For this review, take the finished solid that the model builds, in its own axes (mm). Give positions to 0.01 mm unless a question says otherwise; leave off trailing zeros. Loops run counter-clockwise (first coordinate to the right, second up) from the corner with the lowest first, then second, coordinate; pieces in that order, holes last.
Autodesk Inventor part; units mm, degrees
ref_plane "YZ Plane" through (0, 0, 0) normal (1, 0, 0) x (0, 1, 0)
ref_plane "XZ Plane" through (0, 0, 0) normal (0, 1, 0) x (-1, 0, 0)
ref_plane "XY Plane" through (0, 0, 0) normal (0, 0, 1) x (1, 0, 0)
sketch "Sketch1" plane through (0, 0, 0) normal (0, 0, 1) x (1, 0, 0)
  point P0 (0, 0)
sketch "Sketch2" plane through (0, 0, 0) normal (0, 0, 1) x (1, 0, 0)
  circle A0 centre (0, 0) radius 50
  dimension "d0" = 100
extrude "Extrusion1" add sketch "Sketch2" along normal blind 10
sketch "Sketch5" plane through (0, 0, 10) normal (0, 0, 1) x (1, 0, 0)
  circle A0 centre (0, 0) radius 12.5
  line L0 (0, 0) -> (0, 36)
  circle A1 centre (0, 36) radius 4
  dimension "d16" = 36
  dimension "d17" = 8
extrude "Extrusion4" cut sketch "Sketch5" against normal blind 10 contours A1
sketch "Sketch7" plane through (0, 0, 10) normal (0, 0, 1) x (1, 0, 0)
  circle A0 centre (0, 0) radius 5.5
  dimension "d26" = 11
extrude "Extrusion6" cut sketch "Sketch7" against normal blind 10
pattern_circular "Circular Pattern2" count 6 over 360 about axis through (0, 0, 10) along (0, 0, -1) of "Extrusion4"
equation "\"BendRadius\" = Thickness"
equation "\"BendReliefWidth\" = Thickness"
equation "\"BendReliefDepth\" = 0.5 * Thickness"
equation "\"CornerReliefSize\" = 4 * Thickness"
equation "\"MinimumRemnant\" = 2 * Thickness"
equation "\"TransitionRadius\" = BendRadius"
equation "\"JacobiRadiusSize\" = BendRadius"
equation "\"GapSize\" = Thickness"
properties part number "capp"
Q1. Consider section B-B on y = 0. Give the boundary of the cut face in (x, z).
Answers:
outline: (-50, 0) - (-5.5, 0) - (-5.5, 10) - (-50, 10) - close; (5.5, 0) - (50, 0) - (50, 10) - (5.5, 10) - close
Q2. Mouldability with a two-part tool opening along X and no side actions: class faces 1 (the cylindrical face through (-29.33, -21.55, 5.07)), 2 (the cylindrical face through (47.69, -15.02, 4.93)), 3 (the flat face through (-1, -10, 0)), 4 (the cylindrical face through (-1.19, -5.37, 5.07)) as +X half, -X half, draft (parallel to the pull), parting line (faces both ways), or undercut.
Answers:
face 1: undercut
face 2: parting line
face 3: draft
face 4: undercut
Q3. Consider section C-C on y = 19. Give the boundary of the cut face in (x, z).
Answers:
outline: (-46.25, 0) - (-35.05, 0) - (-35.05, 10) - (-46.25, 10) - close; (-27.3, 0) - (27.3, 0) - (27.3, 10) - (-27.3, 10) - close; (35.05, 0) - (46.25, 0) - (46.25, 10) - (35.05, 10) - close
Q4. For pin 1 Ø7 at (x, y) = (0, 36) entering from -Z; pin 2 Ø14.5 at (x, y) = (0, 0) entering from -Z; pin 3 Ø4 at (x, z) = (-17, 2.5) entering from -Y; pin 4 Ø3 at (y, z) = (-9, 8) entering from +X, all flat-tipped, find the tip position at first contact; note any pin that passes through.
Answers:
pin 1: passes through
pin 2: stops at z = 0
pin 3: stops at y = -47.7
pin 4: stops at x = 49.43
Q5. Consider section A-A on x = 0. Give the boundary of the cut face in (y, z), plus the area to 3 significant figures.
Answers:
outline: (-50, 0) - (-40, 0) - (-40, 10) - (-50, 10) - close; (-32, 0) - (-5.5, 0) - (-5.5, 10) - (-32, 10) - close; (5.5, 0) - (32, 0) - (32, 10) - (5.5, 10) - close; (40, 0) - (50, 0) - (50, 10) - (40, 10) - close
area: 730 mm2
Q6. For probe 1 along Y at (x, z) = (0, 6.5); probe 2 along Y at (x, z) = (-1, 7.5); probe 3 along Y at (x, z) = (30, 3), list the stretches that pass through material, from the lowest coordinate up.
Answers:
probe 1: y = -50 to -40, -32 to -5.5, 5.5 to 32, 40 to 50
probe 2: y = -49.99 to -39.87, -32.13 to -5.41, 5.41 to 32.13, 39.87 to 49.99
probe 3: y = -40 to -21.82, -14.18 to 14.18, 21.82 to 40
Q7. Consider section D-D on z = 4.25. Give the boundary of the cut face in (x, y), plus the area to 3 significant figures.
Answers:
outline: circle Ø100 at (0, 0); hole circle Ø8 at (-31.18, -18); hole circle Ø8 at (-31.18, 18); hole circle Ø11 at (0, 0); hole circle Ø8 at (0, -36); hole circle Ø8 at (0, 36); hole circle Ø8 at (31.18, -18); hole circle Ø8 at (31.18, 18)
area: 7,460 mm2
